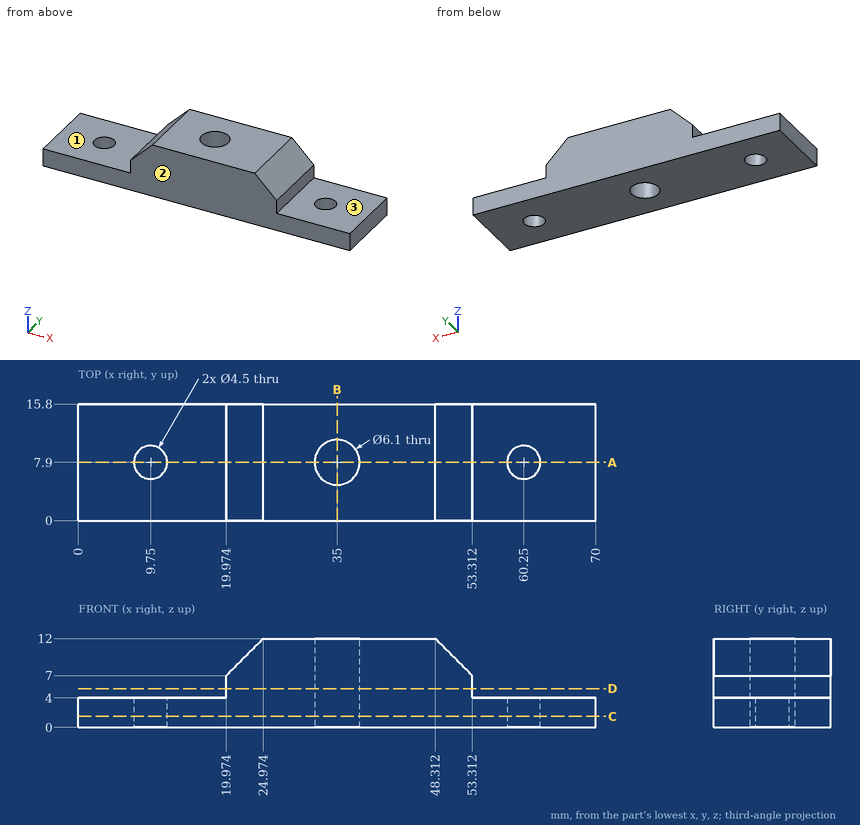
Can you work these out from the drawing? Everything is in mm from the part's minimum corner. A direction names the side the tool comes from. Round coordinates to 2 decimals unless told otherwise and drop trailing zeros. Loops run counter-clockwise (first coordinate to the right, second up) from the corner with the lowest first, then second, coordinate; pieces in that order, holes last. Notation, with made-up numbers: (26.25, 33) -> (34.25, 33) arc R20 ccw to (34.25, 44) -> close; hole circle Ø1 at (62, 44). An arc over 180 degrees is marked (long way). Use CSV: the item, a comma, the result in double quotes.
(1) Suppose I cut it at C-C on z = 1.5. Write out the boundary of the cut face in (x, y), plus the area to 4 significant figures.
Return value:
outline,"(0, 0) -> (70, 0) -> (70, 15.8) -> (0, 15.8) -> close; hole circle Ø4.5 at (9.75, 7.9); hole circle Ø6.1 at (35, 7.9); hole circle Ø4.5 at (60.25, 7.9)"
area,"1,045 mm²"
(2) Suppose I cut it at A-A on y = 7.9. Write out the boundary of the cut face in (x, z).
Return value:
outline,"(0, 0) -> (7.5, 0) -> (7.5, 4) -> (0, 4) -> close; (12, 0) -> (31.95, 0) -> (31.95, 12) -> (24.97, 12) -> (19.97, 7) -> (19.97, 4) -> (12, 4) -> close; (38.05, 0) -> (58, 0) -> (58, 4) -> (53.31, 4) -> (53.31, 7) -> (48.31, 12) -> (38.05, 12) -> close; (62.5, 0) -> (70, 0) -> (70, 4) -> (62.5, 4) -> close"
(3) If I drill on probe 1 along X at (y, z) = (8, 2.25); probe 2 along Y at (x, z) = (60.25, 2.85); probe 3 along Y at (x, z) = (35, 6.25), over which ranges is the centre line in solid material (lowest first)? Write a range as [from, to].
Return value:
probe 1,"x = [0, 7.5], [12, 31.95], [38.05, 58], [62.5, 70]"
probe 2,"y = [0, 5.65], [10.15, 15.8]"
probe 3,"y = [0, 4.85], [10.95, 15.8]"
(4) Will these pins go through, and if not, where does the flat tip stop? pin 1 Ø3 at (y, z) = (4, 6) entering from +X; pin 2 Ø6 at (x, y) = (13, 13.5) entering from +Z; pin 3 Ø0.9 at (y, z) = (6.5, 5.5) entering from -X.
Return value:
pin 1,"stops at x = 53.31"
pin 2,"stops at z = 4"
pin 3,"stops at x = 19.97"
(5) Suppose I cut it at B-B on x = 35. Write out the boundary of the cut face in (y, z).
Return value:
outline,"(0, 0) -> (4.85, 0) -> (4.85, 12) -> (0, 12) -> close; (10.95, 0) -> (15.8, 0) -> (15.8, 12) -> (10.95, 12) -> close"
(6) For the marked faces 1, 2 and 3, which set-ups out of +Z, -Z, +X, -X, +Y, -Y let a thin tool reach every point of the face, with its end or its side?
Return value:
face 1,"+Z, -X, +Y, -Y"
face 2,"+Z, -Z, +X, -X, -Y"
face 3,"+Z, +X, +Y, -Y"
(7) Suppose I cut it at D-D on z = 5.25. Write out the boundary of the cut face in (x, y).
Return value:
outline,"(19.97, 0) -> (53.31, 0) -> (53.31, 15.8) -> (19.97, 15.8) -> close; hole circle Ø6.1 at (35, 7.9)"
